from build123d import *

# Parameters (mm, degrees)
SKETCH1_R           = 22.5
SKETCH1_R_2         = 6.5
BOSS_EXTRUDE1_DEPTH = 12.5
SKETCH2_R           = 6.5
BOSS_EXTRUDE2_DEPTH = 12.5
SKETCH3_R           = 6.5
CUT_EXTRUDE1_DEPTH  = 901.750681353
FILLET1_R           = 13
SKETCH4_W           = 10
SKETCH4_H           = 25.980762113
CUT_EXTRUDE2_DEPTH  = 1021.222656563
SKETCH5_R           = 6.5
CUT_EXTRUDE3_DEPTH  = 5
SKETCH6_W           = 23.820751316
SKETCH6_H           = 10
CUT_EXTRUDE4_DEPTH  = 25
FILLET2_R           = 15


with BuildPart() as part:
    # Sketch1 → Boss-Extrude1 (new, symmetric)
    with BuildSketch(Plane.XY):
        with Locations((434.94970424, -853.401384058)):
            Circle(SKETCH1_R)
        with Locations((434.94970424, -853.401384058)):
            Circle(SKETCH1_R_2, mode=Mode.SUBTRACT)
    extrude(amount=BOSS_EXTRUDE1_DEPTH, both=True)

    # Sketch2 → Boss-Extrude2 (add, symmetric)
    with BuildSketch(Plane.XY):
        with BuildLine():
            Line((440.57470424, -831.615852736), (478.07470424, -841.298311101))
            ThreePointArc((478.07470424, -841.298311101), (486.236797951, -848.030023379), (486.312946026, -858.609717392))
            Line((486.312946026, -858.609717392), (474.94970424, -883.401384058))
            Line((474.94970424, -883.401384058), (469.220338634, -895.901384058))
            Line((469.220338634, -895.901384058), (394.94970424, -895.901384058))
            Line((394.94970424, -895.901384058), (394.94970424, -870.901384058))
            Line((394.94970424, -870.901384058), (416.598084064, -840.383395085))
            ThreePointArc((416.598084064, -840.383395085), (427.222533672, -832.269871216), (440.57470424, -831.615852736))
        make_face()
        with Locations((474.94970424, -853.401384058)):
            Circle(SKETCH2_R, mode=Mode.SUBTRACT)
        with Locations((434.94970424, -853.401384058)):
            Circle(SKETCH2_R, mode=Mode.SUBTRACT)
    extrude(amount=BOSS_EXTRUDE2_DEPTH, both=True)

    # Sketch3 → Cut-Extrude1 (cut, through all)
    with BuildSketch(Plane.ZY.offset(-394.94970424)):
        with Locations(Location((0, -883.401384058, 0), (0, 0, 270))):
            Circle(SKETCH3_R)
    extrude(amount=-CUT_EXTRUDE1_DEPTH, mode=Mode.SUBTRACT)

    # Fillet1
    # the kernel refuses this fillet: 13 mm, written as the material it takes off along each edge
    with BuildSketch(Plane(origin=(501.720338634, -895.901384058, -12.5), x_dir=(0, 1, 0), z_dir=(-1, 0, 0))) as fillet1_piece_1:
        with BuildLine():
            CenterArc((FILLET1_R, -FILLET1_R), FILLET1_R, 90, 90)
            Line((0, -FILLET1_R), (0, 0))
            Line((0, 0), (FILLET1_R, 0))
        make_face()
    extrude(amount=139.270634394, mode=Mode.SUBTRACT)
    with BuildSketch(Plane(origin=(501.720338634, -895.901384058, 12.5), x_dir=(0, 1, 0), z_dir=(-1, 0, 0))) as fillet1_piece_2:
        with BuildLine():
            CenterArc((FILLET1_R, FILLET1_R), FILLET1_R, 180, 90)
            Line((0, FILLET1_R), (0, 0))
            Line((0, 0), (FILLET1_R, 0))
        make_face()
    extrude(amount=139.270634394, mode=Mode.SUBTRACT)

    # Sketch4 → Cut-Extrude2 (cut, through all)
    with BuildSketch(Plane.XY.offset(12.5)):
        with Locations((458.44970424, -882.901384059)):
            Rectangle(SKETCH4_W, SKETCH4_H)
    extrude(amount=-CUT_EXTRUDE2_DEPTH, mode=Mode.SUBTRACT)

    # Sketch5 → Cut-Extrude3 (cut, symmetric)
    with BuildSketch(Plane.XY):
        with BuildLine():
            Line((470.959579505, -839.461193794), (455.767141872, -835.538523265))
            Line((455.767141872, -835.538523265), (460.847639703, -856.775072808))
            ThreePointArc((460.847639703, -856.775072808), (487.47066386, -860.7140833), (470.959579505, -839.461193794))
        make_face()
        with Locations((474.94970424, -853.401384058)):
            Circle(SKETCH5_R, mode=Mode.SUBTRACT)
    extrude(amount=CUT_EXTRUDE3_DEPTH, both=True, mode=Mode.SUBTRACT)

    # Sketch6 → Cut-Extrude4 (cut)
    with BuildSketch(Plane(origin=(-173.766227741, -672.993706172, 0), x_dir=(0.9682458365518545, -0.24999999999999928, 0), z_dir=(0.24999999999999928, 0.9682458365518545, 0))):
        with Locations((672.317952287, 0)):
            Rectangle(SKETCH6_W, SKETCH6_H)
    extrude(amount=-CUT_EXTRUDE4_DEPTH, mode=Mode.SUBTRACT)

    # Fillet2
    # the kernel refuses this fillet: 15 mm, written as the material it takes off along each edge
    with BuildSketch(Plane(origin=(481.95399382, -868.119828339, 5), x_dir=(-0.9682458365518494, 0.2500000000000187, 0), z_dir=(0, 0, -1))) as fillet2_piece_1:
        with BuildLine():
            CenterArc((16.462547076, -6.840323223), FILLET2_R, 152.869318281, 37.277487885)
            Line((1.697153218, -9.482887166), (0, 0))
            Line((0, 0), (3.113016066, 0))
        make_face()
    extrude(amount=10, mode=Mode.SUBTRACT)


solid = part.part
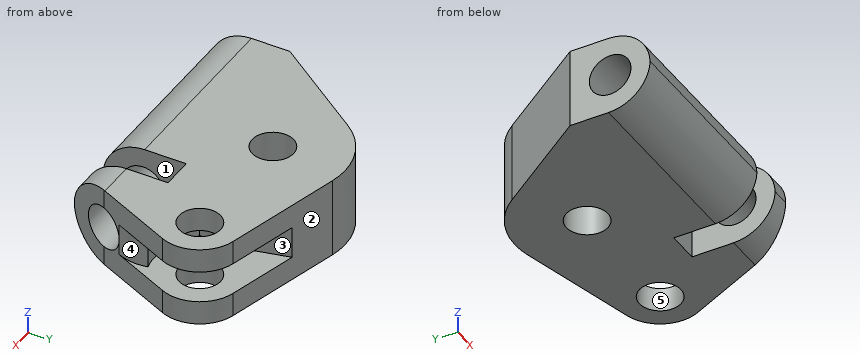
For this review, take the finished solid that the model builds, in its own axes (mm). Face numbers are marked on the shaded views. A direction names the side the tool comes from. Give positions to 0.01 mm unless a question says otherwise; leave off trailing zeros. Loops run counter-clockwise (first coordinate to the right, second up) from the corner with the lowest first, then second, coordinate; pieces in that order, holes last.
Item 1: Take a section at C-C, the plane x = 414.5. State the section outline as (y, z) points, and give its area (3 significant figures).
Item 2: Take a section at A-A, the plane z = 2.5. State the section outline as (x, y) points.
Item 3: For line 1 along X through (y, z) = (-871, 0.5); line 2 along Z through (x, y) = (470, -863); line 3 along Y through (x, z) = (469.5, 6), list the stretches that pass through material, from the lowest coordinate up.
Item 4: Take a section at D-D, the plane z = 8.25. State the section outline as (x, y) points, and give its area (3 significant figures).
Item 5: Tool access review of the marked faces 1 and 2: name each direction out of +Z, -Z, +X, -X, +Y, -Y from which nothing blocks a thin tool from reaching the whole face with its end or side.
Item 6: Insertion check: pin 1 (10.5 mm diameter, centred on x = 434.95, y = -853.4, fed in from -Z); pin 2 (15 mm diameter, centred on y = -883.4, z = 0, fed in from +X); pin 3 (6 mm diameter, centred on y = -857.5, z = -7.5, fed in from +X); pin 4 (3 mm diameter, centred on x = 458.5, z = -4.5, fed in from -Y). Each pin has a flat end and moves straight along its axis. Give the tip position at first contact, or say it passes through.
Item 7: Take a section at B-B, the plane y = -886.5. State the section outline as (x, z) points, and give its area (3 significant figures).
Item 8: Draft analysis for pull direction Y (two halves, no side actions). For the marked faces 3, 4 and 5, state which applies: +Y half, -Y half, draft (parallel to the pull), parting line (faces both ways), or undercut.
Calculated:
1. outline: (-895.89, 0) arc R13 ccw to (-882.9, -12.5) - (-843.34, -12.5) - (-843.34, 12.5) - (-882.9, 12.5) arc R13 ccw to start; hole circle Ø13 at (-883.4, 0)
1. area: 1,110 mm2
2. outline: (394.95, -895.55) - (453.45, -895.55) - (453.45, -889.4) - (394.95, -889.4) - close; (394.95, -877.4) - (453.45, -877.4) - (453.45, -869.91) - (463.45, -869.91) - (463.45, -877.4) - (477.7, -877.4) - (477.94, -876.88) arc R15 ccw to (478.94, -867.34) arc R14.5 cw to (464.71, -863.67) - (459.42, -862.3) - (460.85, -856.78) - (455.77, -835.54) - (440.57, -831.62) arc R22.5 ccw to (416.6, -840.38) - (394.95, -870.9) - close; (463.45, -895.55) - (469.38, -895.55) - (472.2, -889.4) - (463.45, -889.4) - close; hole circle Ø13 at (434.95, -853.4)
3. line 1: x = 394.95 to 453.45, 463.45 to 479.3
3. line 2: z = -12.5 to -5, 5 to 12.5
3. line 3: y = -894.16 to -885.9, -880.9 to -856.94, -849.86 to -839.08
4. outline: (394.95, -892.52) - (453.45, -892.52) - (453.45, -869.91) - (463.45, -869.91) - (463.45, -892.52) - (470.77, -892.52) - (486.31, -858.61) arc R12.5 ccw to (478.07, -841.3) - (440.57, -831.62) arc R22.5 ccw to (416.6, -840.38) - (394.95, -870.9) - close; hole circle Ø13 at (434.95, -853.4); hole circle Ø13 at (474.95, -853.4)
4. area: 3,980 mm2
5. face 1: +Z, -Z, -Y
5. face 2: +Z, -Z, +X, +Y
6. pin 1: passes through
6. pin 2: stops at x = 478.35
6. pin 3: stops at x = 487.4
6. pin 4: stops at y = -869.91
7. outline: (394.95, -11.99) - (453.45, -11.99) - (453.45, -5.71) - (394.95, -5.71) - close; (394.95, 5.71) - (453.45, 5.71) - (453.45, 11.99) - (394.95, 11.99) - close; (463.45, -11.99) - (473.53, -11.99) - (473.53, -5.71) - (463.45, -5.71) - close; (463.45, 5.71) - (473.53, 5.71) - (473.53, 11.99) - (463.45, 11.99) - close
7. area: 861 mm2
8. face 3: +Y half
8. face 4: parting line
8. face 5: undercut
